Build history of the part. All positions in model axes, mm. Face numbers are marked on the shaded views. A direction names the side the tool comes from. Give positions to 0.01 mm unless a question says otherwise; leave off trailing zeros. Order: outer loops, then holes, each group sorted by start corner. A loop starts at its lowest first (then second) coordinate and runs counter-clockwise, first axis right, second up. Notation, with made-up numbers: (-11, 20) - (-1, 20) arc R23 ccw to (-1, 42) - close; hole circle Ø5 at (-9, 57.5). An arc over 180 degrees is marked (long way). Write each question's results on one line, items separated by ' | '. Start each with the question number.
1) Tool access for the marked faces 1 and 2: list every direction of +Z, -Z, +X, -X, +Y, -Y with a clear straight run to the whole face (end or side of a thin tool).
2) Cut at A-A on x = 0. List the corners of the cut face in (y, z).
3) Drop flat-ended pins along their axis: pin 1 Ø4 at (x, z) = (2, 12.5) entering from +Y; pin 2 Ø2 at (x, z) = (-1.5, 0.5) entering from -Y; pin 3 Ø3 at (y, z) = (0.5, 26) entering from -X. Give the stop position or say it passes through.
4) Drill centre lines: line 1 along Z through (x, y) = (-2, -2.75); line 2 along Z through (x, y) = (0.25, 0.5); line 3 along Y through (x, z) = (0, 19). Where is each one in solid material? Low to high. Write a range as from..to.
5) Cut at C-C on y = -3. List the corners of the cut face in (x, z).
6) Cut at B-B on z = 23.5. List the corners of the cut face in (x, y), plus the area to 3 significant figures.
from build123d import *

# Parameters (mm, degrees)
F_01_START                  = -2.8
S01_LOW_SOCKET_HEAD_R       = 3.5
F_01_LOW_SOCKET_HEAD_DEPTH  = 2.8
S02_NOMINAL_M4_SHANK_R      = 2
F_02_NOMINAL_M4_SHANK_DEPTH = 30
F_03_START                  = -2.9
F_03_HEX_DRIVE_RECESS_DEPTH = 1.65


with BuildPart() as part:
    # S01 - Low socket head → 01 - Low socket head (new body)
    with BuildSketch(Plane.XY.offset(F_01_START)):
        Circle(S01_LOW_SOCKET_HEAD_R)
    extrude(amount=F_01_LOW_SOCKET_HEAD_DEPTH)

    # S02 - Nominal M4 shank → 02 - Nominal M4 shank (add)
    with BuildSketch(Plane.XY):
        Circle(S02_NOMINAL_M4_SHANK_R)
    extrude(amount=F_02_NOMINAL_M4_SHANK_DEPTH)

    # S03 - Hex drive recess → 03 - Hex drive recess (cut)
    with BuildSketch(Plane.XY.offset(F_03_START)):
        Polygon((1.443375673, 0), (0.721687836, 1.25), (-0.721687836, 1.25), (-1.443375673, 0), (-0.721687836, -1.25), (0.721687836, -1.25), align=None)
    extrude(amount=F_03_HEX_DRIVE_RECESS_DEPTH, mode=Mode.SUBTRACT)


solid = part.part
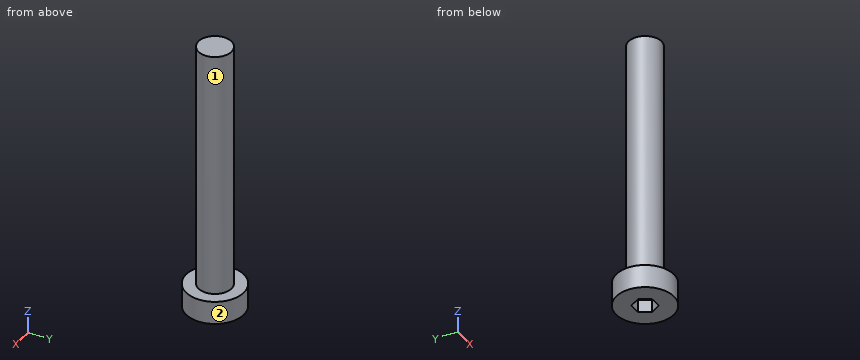
Results:
1) face 1: +Z | face 2: +Z, -Z
2) outline: (-3.5, -2.8) - (-1.25, -2.8) - (-1.25, -1.25) - (1.25, -1.25) - (1.25, -2.8) - (3.5, -2.8) - (3.5, 0) - (2, 0) - (2, 30) - (-2, 30) - (-2, 0) - (-3.5, 0) - close
3) pin 1: y = 2 | pin 2: y = -3.44 | pin 3: x = -2
4) line 1: -2.8..0 | line 2: -1.25..30 | line 3: -2..2
5) outline: (-1.8, -2.8) - (1.8, -2.8) - (1.8, 0) - (-1.8, 0) - close
6) outline: circle Ø4 at (0, 0) | area: 12.6 mm^2
